from build123d import *

# Parameters (mm, degrees)
SKETCH_1_W          = 111
SKETCH_1_H          = 35
SKETCH_1_R          = 1.8
EXTRUDE_1_DEPTH     = 4.75
SKETCH_2_W          = 4
SKETCH_2_H          = 35
EXTRUDE_2_DEPTH     = 15.5
SKETCH_3_W          = 4.5
SKETCH_3_H          = 35
EXTRUDE_3_DEPTH     = 14
SKETCH_4_W          = 4.5
SKETCH_4_H          = 35
EXTRUDE_4_DEPTH     = 14
FILLET_1_R          = 5
FILLET_2_R          = 1
SKETCH_5_W          = 20
SKETCH_5_H          = 2
CUT_EXTRUDE_1_DEPTH = 1
CUT_EXTRUDE_2_DEPTH = 200
SKETCH_8_W          = 33.5
SKETCH_8_H          = 25
SKETCH_8_W_2        = 38
CUT_EXTRUDE_3_DEPTH = 1000
FILLET_8_R          = 10
FILLET_9_R          = 4
FILLET_10_R         = 0.5


with BuildPart() as part:
    # ｽｹｯﾁ1 → ﾎﾞｽ - 押し出し1 (new body)
    with BuildSketch(Plane.XY):
        with Locations((0, -98.5)):
            Rectangle(SKETCH_1_W, SKETCH_1_H)
        with Locations((25, -111)):
            Circle(SKETCH_1_R, mode=Mode.SUBTRACT)
        with Locations((15, -111)):
            Circle(SKETCH_1_R, mode=Mode.SUBTRACT)
        with Locations((-15, -111)):
            Circle(SKETCH_1_R, mode=Mode.SUBTRACT)
        with Locations((-25, -111)):
            Circle(SKETCH_1_R, mode=Mode.SUBTRACT)
    extrude(amount=EXTRUDE_1_DEPTH)

    # ｽｹｯﾁ2 → ﾎﾞｽ - 押し出し2 (add)
    with BuildSketch(Plane.XY.offset(4.75)):
        with Locations((39.5, -98.5)):
            Rectangle(SKETCH_2_W, SKETCH_2_H)
        with Locations((-39.5, -98.5)):
            Rectangle(SKETCH_2_W, SKETCH_2_H)
    extrude(amount=EXTRUDE_2_DEPTH)

    # ｽｹｯﾁ3 → ﾎﾞｽ - 押し出し3 (add)
    with BuildSketch(Plane(origin=(41.5, 0, 0), x_dir=(0, 0, -1), z_dir=(1, 0, 0))):
        with Locations((-18, -98.5)):
            Rectangle(SKETCH_3_W, SKETCH_3_H)
    extrude(amount=EXTRUDE_3_DEPTH)

    # ｽｹｯﾁ4 → ﾎﾞｽ - 押し出し4 (add)
    with BuildSketch(Plane.ZY.offset(41.5)):
        with Locations((18, -98.5)):
            Rectangle(SKETCH_4_W, SKETCH_4_H)
    extrude(amount=EXTRUDE_4_DEPTH)

    # ﾌｨﾚｯﾄ1
    fillet_1_edges = [part.edges().sort_by_distance(p)[0] for p in [
        (37.5, -98.5, 4.75),
        (-37.5, -98.5, 4.75),
    ]]
    fillet(fillet_1_edges, radius=FILLET_1_R)

    # ﾌｨﾚｯﾄ2
    fillet_2_edges = [part.edges().sort_by_distance(p)[0] for p in [
        (37.5, -98.5, 20.25),
        (-37.5, -98.5, 20.25),
        (-55.5, -98.5, 0),
        (55.5, -98.5, 20.25),
        (55.5, -98.5, 0),
        (-55.5, -98.5, 20.25),
    ]]
    fillet(fillet_2_edges, radius=FILLET_2_R)

    # ｽｹｯﾁ5 → ｶｯﾄ - 押し出し1 (cut)
    with BuildSketch(Plane(origin=(0, -81, 0), x_dir=(1, 0, 0), z_dir=(0, 1, 0))):
        with Locations((0, -3.75)):
            Rectangle(SKETCH_5_W, SKETCH_5_H)
    extrude(amount=-CUT_EXTRUDE_1_DEPTH, mode=Mode.SUBTRACT)

    # ｽｹｯﾁ6 → ｶｯﾄ - 押し出し2 (cut)
    with BuildSketch(Plane(origin=(0, -81, 0), x_dir=(1, 0, 0), z_dir=(0, 1, 0))):
        Polygon((-55.5, -4.75), (-48.5, -4.75), (-55.5, -3.25), align=None)
        Polygon((-41.5, -4.75), (-41.5, -3.25), (-48.5, -4.75), align=None)
        Polygon((-41.5, -15.75), (-48.5, -15.75), (-41.5, -17.25), align=None)
        Polygon((-55.5, -17.25), (-48.5, -15.75), (-55.5, -15.75), align=None)
        Polygon((55.5, -4.75), (55.5, -3.25), (48.5, -4.75), align=None)
        Polygon((41.5, -4.75), (48.5, -4.75), (41.5, -3.25), align=None)
        Polygon((55.5, -15.75), (48.5, -15.75), (55.5, -17.25), align=None)
        Polygon((41.5, -15.75), (41.5, -17.25), (48.5, -15.75), align=None)
    extrude(amount=-CUT_EXTRUDE_2_DEPTH, mode=Mode.SUBTRACT)

    # ｽｹｯﾁ8 → ｶｯﾄ - 押し出し3 (cut)
    with BuildSketch(Plane(origin=(0, 0, 0), x_dir=(-1, 0, 0), z_dir=(0, 0, -1))):
        with Locations((-47.75, -103.5)):
            Rectangle(SKETCH_8_W, SKETCH_8_H)
        with Locations((0, -93.5)):
            Rectangle(SKETCH_8_W_2, SKETCH_8_H)
        with Locations((47.75, -103.5)):
            Rectangle(SKETCH_8_W, SKETCH_8_H)
    extrude(amount=-CUT_EXTRUDE_3_DEPTH, mode=Mode.SUBTRACT)

    # ﾌｨﾚｯﾄ8
    fillet_8_edges = [part.edges().sort_by_distance(p)[0] for p in [
        (-31, -91, 2.375),
        (31, -91, 2.375),
        (-19, -106, 2.375),
        (19, -106, 2.375),
    ]]
    fillet(fillet_8_edges, radius=FILLET_8_R)

    # ﾌｨﾚｯﾄ9
    fillet_9_edges = [part.edges().sort_by_distance(p)[0] for p in [
        (31, -116, 2.375),
        (-31, -116, 2.375),
        (19, -81, 2.375),
        (-19, -81, 2.375),
    ]]
    fillet(fillet_9_edges, radius=FILLET_9_R)

    # ﾌｨﾚｯﾄ10
    fillet_10_edges = [part.edges().sort_by_distance(p)[0] for p in [
        (-55.5, -86, 17.25),
        (48.5, -86, 15.75),
        (55.5, -86, 17.25),
        (48.5, -86, 4.75),
        (41.5, -86, 3.25),
        (-48.5, -86, 15.75),
        (-41.5, -86, 17.25),
        (-41.5, -86, 3.25),
        (-48.5, -86, 4.75),
        (-55.5, -86, 3.25),
        (55.5, -86, 3.25),
        (41.5, -86, 17.25),
    ]]
    fillet(fillet_10_edges, radius=FILLET_10_R)


solid = part.part
Design review of the part built by this model. Coordinates are the model's own, in mm. A direction names the side the tool comes from. Round coordinates to 2 decimals unless told otherwise and drop trailing zeros. Write each loop counter-clockwise with the first axis right and the second up, starting at its lowest first coordinate (ties: lowest second). Pieces come first, ordered by that corner, then holes. Notation, with made-up numbers: (5.25, 87.5) - (55.25, 87.5) arc R20 cw to (55.25, 100.5) - close; hole circle Ø2 at (29.5, 44). An arc over 180 degrees is marked (long way). Use a Markdown table: item, result. Add a question column.
1. Mouldability with a two-part tool opening along Y and no side actions: class faces 4 (the face through (-36.874, -91.891, 5.767)), 5 (the face through (-14.169, -112.597, 2.342)), 6 (the face through (20.141, -82.203, 2.408)), 7 (the face through (37.5, -86, 14)) as +Y half, -Y half, draft (parallel to the pull), parting line (faces both ways), or undercut.
2. Wall thickness on probe 1 along X at (y, z) = (-111, 3.3); probe 2 along Y at (x, z) = (-25, 2.55); probe 3 along X at (y, z) = (-108, 2.5): over which ranges is each line inside the solid? List them lowest first.
3. We need section A-A (x = 25). State the section outline as (y, z) points, then the cut area to 3 significant figures.
4. Clearance check with flat-ended pins moving along their axes: pin 1 (12 mm diameter, centred on x = -26.5, z = 11.5, fed in from +Y); pin 2 (2.5 mm diameter, centred on x = -1.5, z = 2.5, fed in from +Y); pin 3 (2 mm diameter, centred on x = -11, z = 4, fed in from +Y); pin 4 (11 mm diameter, centred on y = -86.5, z = 8.5, fed in from +X). State where each tip first meets the part, or that it passes through.
5. We need section C-C (z = 8). State the section outline as (x, y) points, then the cut area to 3 significant figures.
6. We need section B-B (y = -111). State the section outline as (x, z) points.
7. For faces 1 (the face through (-16.15, -102.99, 2.41)), 2 (the face through (-48, -91, 3)), 3 (the face through (-52, -86, 4)), list the 3-axis set-ups (+Z, -Z, +X, -X, +Y, -Y) from which the entire face can be reached by the end or side of a thin tool; tool diameter is ignored.
8. We need section D-D (y = -94.5). State the section outline as (x, z) points.
Output:
| question | item | result |
|---|---|---|
| 1 | face 4 | -Y half |
| 1 | face 5 | undercut |
| 1 | face 6 | +Y half |
| 1 | face 7 | draft |
| 2 | probe 1 | x = -31 to -26.8, -23.2 to -16.8, -13.2 to 13.2, 16.8 to 23.2, 26.8 to 31 |
| 2 | probe 2 | y = -116 to -112.8, -109.2 to -81 |
| 2 | probe 3 | x = -31 to 31 |
| 3 | outline | (-116, 0) - (-112.8, 0) - (-112.8, 4.75) - (-116, 4.75) - close; (-109.2, 0) - (-81, 0) - (-81, 4.75) - (-109.2, 4.75) - close |
| 3 | area | 149 mm2 |
| 4 | pin 1 | passes through |
| 4 | pin 2 | stops at y = -106 |
| 4 | pin 3 | stops at y = -105.54 |
| 4 | pin 4 | stops at x = 55.48 |
| 5 | outline | (-41.5, -91) - (-41, -91) arc R10 cw to (-37.18, -91.76) - (-37.18, -81) - (-41.5, -81) - close; (37.18, -91.76) arc R10 cw to (41, -91) - (41.5, -91) - (41.5, -81) - (37.18, -81) - close |
| 5 | area | 88.2 mm2 |
| 6 | outline | (-31, 0) - (-26.8, 0) - (-26.8, 4.75) - (-31, 4.75) - close; (-23.2, 0) - (-16.8, 0) - (-16.8, 4.75) - (-23.2, 4.75) - close; (-13.2, 0) - (13.2, 0) - (13.2, 4.75) - (-13.2, 4.75) - close; (16.8, 0) - (23.2, 0) - (23.2, 4.75) - (16.8, 4.75) - close; (26.8, 0) - (31, 0) - (31, 4.75) - (26.8, 4.75) - close |
| 7 | face 1 | +Z, -Z, +Y |
| 7 | face 2 | +Z, -Z, -X, -Y |
| 7 | face 3 | -X, +Y, -Y |
| 8 | outline | (-33.4, 0) - (-19, 0) - (-19, 4.75) - (-32.5, 4.75) arc R5 cw to (-33.4, 4.83) - close; (19, 0) - (33.4, 0) - (33.4, 4.83) arc R5 cw to (32.5, 4.75) - (19, 4.75) - close |
